```python
from build123d import *

# Parameters (mm, degrees)
SKETCH_1_R               = 3.5
EXTRUDE_1_DEPTH          = 60
FILLET_1_R               = 1.5
SKETCH_2_R               = 6.25
CUT_EXTRUDE_1_DEPTH      = 20
CUT_EXTRUDE_START        = -20
SKETCH_3_R               = 6.25
CUT_EXTRUDE_2_DEPTH      = 20
SKETCH_5_W               = 8
SKETCH_5_H               = 0.75
CUT_EXTRUDE_4_DEPTH      = 62
FILLET_2_R               = 1
SKETCH_7_W               = 8
SKETCH_7_H               = 30
EXTRUDE_2_DEPTH          = 2
SKETCH_6_R               = 1.25
CUT_EXTRUDE_5_DEPTH      = 62
SKETCH_8_R               = 1.25
CUT_EXTRUDE_6_DEPTH      = 5
CUT_EXTRUDE_9_DEPTH      = 5
CUT_EXTRUDE_9_DEPTH_BACK = 8


with BuildPart() as part:
    # 草图1 → 凸台-拉伸1 (new body)
    with BuildSketch(Plane.XY):
        Polygon((-20, -7.5), (-20, 9), (20, 9), (20, -7.5), (0, -7.5), align=None)
        with Locations((-10, 0)):
            Circle(SKETCH_1_R, mode=Mode.SUBTRACT)
        with Locations((10, 0)):
            Circle(SKETCH_1_R, mode=Mode.SUBTRACT)
    extrude(amount=EXTRUDE_1_DEPTH)

    # 圆角1
    fillet_1_edges = [part.edges().sort_by_distance(p)[0] for p in [
        (-20, -7.5, 30),
        (-20, 9, 30),
        (20, 9, 30),
        (20, -7.5, 30),
    ]]
    fillet(fillet_1_edges, radius=FILLET_1_R)

    # 草图2 → 切除-拉伸1 (cut)
    with BuildSketch(Plane.XY.offset(60)):
        with Locations((10, 0)):
            Circle(SKETCH_2_R)
        with Locations((-10, 0)):
            Circle(SKETCH_2_R)
    extrude(amount=-CUT_EXTRUDE_1_DEPTH, mode=Mode.SUBTRACT)

    # 草图3 → 切除-拉伸2 (cut)
    with BuildSketch(Plane(origin=(0, 0, 0), x_dir=(-1, 0, 0), z_dir=(0, 0, -1)).offset(CUT_EXTRUDE_START)):
        with Locations(Location((-10, 0, 0), (0, 0, 180))):
            Circle(SKETCH_3_R)
        with Locations(Location((10, 0, 0), (0, 0, 180))):
            Circle(SKETCH_3_R)
    extrude(amount=CUT_EXTRUDE_2_DEPTH, mode=Mode.SUBTRACT)

    # 草图5 → 切除-拉伸4 (cut)
    with BuildSketch(Plane(origin=(0, 0, 0), x_dir=(-1, 0, 0), z_dir=(0, 0, -1))):
        Polygon((0, -5), (4, -5), (4, -9), (-4, -9), (-4, -5), align=None)
        with Locations((0, 8.625)):
            Rectangle(SKETCH_5_W, SKETCH_5_H)
    extrude(amount=-CUT_EXTRUDE_4_DEPTH, mode=Mode.SUBTRACT)

    # 圆角2
    fillet_2_edges = [part.edges().sort_by_distance(p)[0] for p in [
        (4, -7.5, 30),
        (-4, -7.5, 30),
        (4, -5, 30),
        (-4, -5, 30),
    ]]
    fillet(fillet_2_edges, radius=FILLET_2_R)

    # 草图7 → 凸台-拉伸2 (add)
    with BuildSketch(Plane(origin=(0, 9, 0), x_dir=(1, 0, 0), z_dir=(0, 1, 0))):
        with Locations((0, -30)):
            Rectangle(SKETCH_7_W, SKETCH_7_H)
    extrude(amount=-EXTRUDE_2_DEPTH)

    # 草图6 → 切除-拉伸5 (cut)
    with BuildSketch(Plane(origin=(0, 9, 0), x_dir=(1, 0, 0), z_dir=(0, 1, 0))):
        with Locations(Location((0, -26.5, 0), (0, 0, 270))):
            Circle(SKETCH_6_R)
        with Locations(Location((0, -33.5, 0), (0, 0, 270))):
            Circle(SKETCH_6_R)
    extrude(amount=-CUT_EXTRUDE_5_DEPTH, mode=Mode.SUBTRACT)

    # 草图8 → 切除-拉伸6 (cut)
    with BuildSketch(Plane(origin=(0, 9, 0), x_dir=(1, 0, 0), z_dir=(0, 1, 0))):
        with Locations(Location((-10.5, -23, 0), (0, 0, 270))):
            Circle(SKETCH_8_R)
        with Locations(Location((-10.5, -37, 0), (0, 0, 270))):
            Circle(SKETCH_8_R)
    extrude(amount=-CUT_EXTRUDE_6_DEPTH, mode=Mode.SUBTRACT)

    # 草图9 → 切除-拉伸9 (cut, two sides: drawn at the far end of the back side and taken through both)
    with BuildSketch(Plane.XZ.offset(5).offset(-CUT_EXTRUDE_9_DEPTH_BACK)):
        with BuildLine():
            Line((2.474873734, 28.974873734), (2.474873734, 31.025126266))
            ThreePointArc((2.474873734, 31.025126266), (0, 37), (-2.474873734, 31.025126266))
            Line((-2.474873734, 31.025126266), (-2.474873734, 28.974873734))
            ThreePointArc((-2.474873734, 28.974873734), (0, 23), (2.474873734, 28.974873734))
        make_face()
    extrude(amount=CUT_EXTRUDE_9_DEPTH + CUT_EXTRUDE_9_DEPTH_BACK, mode=Mode.SUBTRACT)


solid = part.part
```
Read the model definition and answer for the solid it produces. Units are mm, in the model's axes. A direction names the side the tool comes from. Coordinates: 2 decimals unless noted, no trailing zeros. Write each loop counter-clockwise with the first axis right and the second up, starting at its lowest first coordinate (ties: lowest second). Pieces come first, ordered by that corner, then holes. Notation, with made-up numbers: (-2, 55.5) -> (18, 55.5) arc R31 ccw to (18, 89.5) -> close; hole circle Ø2 at (38, -25.75). An arc over 180 degrees is marked (long way). Write item = value, one per line.
(1) Given pin 1 Ø5 at (x, z) = (1, 44) entering from -Y; pin 2 Ø4 at (x, y) = (7.5, 1) entering from -Z; pin 3 Ø6.5 at (x, z) = (0, 51) entering from +Y, each flat-ended and moving along its own axis, determine where each tip first touches the part or whether it passes through.
From the geometry:
pin_1 = -5.13
pin_2 = 20
pin_3 = 8.25
(2) Section C-C on x = 10 is taken. Write down the section's boundary in (y, z), plus the area to 3 significant figures.
From the geometry:
outline = (-7.5, 0) -> (-6.25, 0) -> (-6.25, 20) -> (-3.5, 20) -> (-3.5, 40) -> (-6.25, 40) -> (-6.25, 60) -> (-7.5, 60) -> close; (3.5, 20) -> (6.25, 20) -> (6.25, 0) -> (9, 0) -> (9, 60) -> (6.25, 60) -> (6.25, 40) -> (3.5, 40) -> close
area = 350 mm2
(3) Which of the six approach directions +Z, -Z, +X, -X, +Y, -Y give full straight-line access (tool end or side, diameter ignored) to faces 1 (the face through (15.96, 1.88, 50.14)), 2 (the face through (0, 8.25, 7)), 3 (the face through (2.475, -1, 30)), 4 (the face through (-10, 4, 37))?
From the geometry:
face_1 = +Z
face_2 = -Z, +Y
face_3 = -Y
face_4 = +Y
(4) Section A-A on z = 26.5 is taken. Write down the section's boundary in (x, y).
From the geometry:
outline = (-20, -6) arc R1.5 ccw to (-18.5, -7.5) -> (-5, -7.5) arc R1 ccw to (-4, -6.5) -> (-4, -6) arc R1 cw to (-3.5, -5.13) -> (-3.5, 3) -> (-1.25, 3) -> (-1.25, 9) -> (-18.5, 9) arc R1.5 ccw to (-20, 7.5) -> close; (1.25, 3) -> (3.5, 3) -> (3.5, -5.13) arc R1 cw to (4, -6) -> (4, -6.5) arc R1 ccw to (5, -7.5) -> (18.5, -7.5) arc R1.5 ccw to (20, -6) -> (20, 7.5) arc R1.5 ccw to (18.5, 9) -> (1.25, 9) -> close; hole circle Ø7 at (-10, 0); hole circle Ø7 at (10, 0)
(5) Section B-B on y = 0 is taken. Count the separate pieces of the cut face and the enclosed holes in it, plus the area to 3 significant figures.
From the geometry:
separate_pieces = 3
enclosed_holes = 1
area = 1,040 mm2
(6) Straight lines are drawn through the part: L1, parallel to X at y = 5.75, z = 33.5; L2, parallel to X at y = 2.25, z = 50; L3, parallel to X at y = -3.25, z = 58. For each, find the intervals that lie inside material, in ascending order. Write a range as from..to.
From the geometry:
L1 = -20..-1.25, 1.25..20
L2 = -20..-15.83, -4.17..4.17, 15.83..20
L3 = -20..-15.34, -4.66..4.66, 15.34..20
(7) Section D-D on z = 48 is taken. Write down the section's boundary in (x, y).
From the geometry:
outline = (-20, -6) arc R1.5 ccw to (-18.5, -7.5) -> (-5, -7.5) arc R1 ccw to (-4, -6.5) -> (-4, -6) arc R1 cw to (-3, -5) -> (3, -5) arc R1 cw to (4, -6) -> (4, -6.5) arc R1 ccw to (5, -7.5) -> (18.5, -7.5) arc R1.5 ccw to (20, -6) -> (20, 7.5) arc R1.5 ccw to (18.5, 9) -> (4, 9) -> (4, 8.25) -> (-4, 8.25) -> (-4, 9) -> (-18.5, 9) arc R1.5 ccw to (-20, 7.5) -> close; hole circle Ø12.5 at (-10, 0); hole circle Ø12.5 at (10, 0)
(8) For a pull along X with two mould halves and no side action, classify faces 5 (the face through (0, -1, 23)), 6 (the face through (13, 3, 20)), 7 (the face through (-19.57, -7.05, 30.42)), 8 (the face through (19.55, -7.07, 30.42)) as +X half, -X half, draft (parallel to the pull), parting line (faces both ways), or undercut.
From the geometry:
face_5 = undercut
face_6 = undercut
face_7 = -X half
face_8 = +X half
